Geometry: see drawing. Coordinates: mm, zero at the bounding-box minimum. A direction names the side the tool comes from. Give positions to 0.01 mm unless a question says otherwise; leave off trailing zeros. Write each loop counter-clockwise with the first axis right and the second up, starting at its lowest first coordinate (ties: lowest second). Pieces come first, ordered by that corner, then holes.
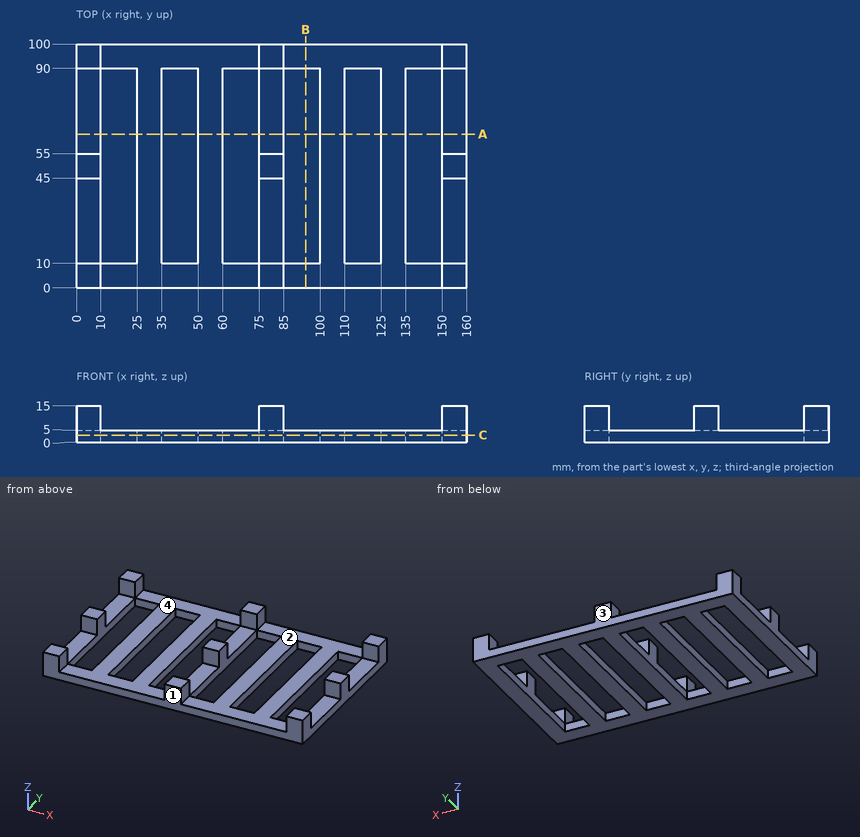
Q1. Section B-B, the plane x = 94. Return the cut outline in (y, z).
Q2. Pin query (flat end, axial travel): pin 1 (5 mm diameter, centred on x = 82, y = 31, fed in from +Z); pin 2 (4 mm diameter, centred on x = 112.5, y = 34.5, fed in from +Z). Return the tip coordinate at first contact, or that it passes through.
Q3. Section A-A, the plane y = 63. Return the cut outline in (x, z), then the cut area to 3 significant figures.
Q4. Mould query, pull axis X, two halves, no side actions, for the marked faces 3 and 4. Classes: +X half, -X half, draft (parallel to the pull), parting line (faces both ways), or undercut.
Q5. Access query for the marked faces 1 and 2. Directions: +Z, -Z, +X, -X, +Y, -Y. A direction counts if a zero-diameter tool reaches every point of the face in a straight line with its end or side. Return the directions, or none.
Q6. Section C-C, the plane z = 3. Return the cut outline in (x, y).
Q7. Material intervals for line 1 along X through (y, z) = (45.5, 6); line 2 along Y through (x, z) = (110.5, 2.5); line 3 along Z through (x, y) = (69.5, 91.5), sorted ascending.
Solutions:
1. outline: (0, 0) - (10, 0) - (10, 5) - (0, 5) - close; (90, 0) - (100, 0) - (100, 5) - (90, 5) - close
2. pin 1: stops at z = 5
2. pin 2: passes through
3. outline: (0, 0) - (10, 0) - (10, 5) - (0, 5) - close; (25, 0) - (35, 0) - (35, 5) - (25, 5) - close; (50, 0) - (60, 0) - (60, 5) - (50, 5) - close; (75, 0) - (85, 0) - (85, 5) - (75, 5) - close; (100, 0) - (110, 0) - (110, 5) - (100, 5) - close; (125, 0) - (135, 0) - (135, 5) - (125, 5) - close; (150, 0) - (160, 0) - (160, 5) - (150, 5) - close
3. area: 350 mm2
4. face 3: draft
4. face 4: undercut
5. face 1: +Z, -Z, +X, -X, -Y
5. face 2: +Z, +Y, -Y
6. outline: (0, 0) - (160, 0) - (160, 100) - (0, 100) - close; hole (10, 10) - (25, 10) - (25, 90) - (10, 90) - close; hole (35, 10) - (50, 10) - (50, 90) - (35, 90) - close; hole (60, 10) - (75, 10) - (75, 90) - (60, 90) - close; hole (85, 10) - (100, 10) - (100, 90) - (85, 90) - close; hole (110, 10) - (125, 10) - (125, 90) - (110, 90) - close; hole (135, 10) - (150, 10) - (150, 90) - (135, 90) - close
7. line 1: x = 0 to 10, 75 to 85, 150 to 160
7. line 2: y = 0 to 10, 90 to 100
7. line 3: z = 0 to 5
